```python
from build123d import *

# Parameters (mm, degrees)
SALIENTE_EXTRUIR1_DEPTH = 600
CROQUIS2_R              = 1.25
CORTAR_EXTRUIR1_DEPTH   = 41


with BuildPart() as part:
    # Croquis1 → Saliente-Extruir1 (new body)
    with BuildSketch(Plane(origin=(0, 0, 0), x_dir=(0, 0, -1), z_dir=(1, 0, 0))):
        Polygon((-20, 0), (20, 0), (20, 15), (18.5, 15), (-18.5, 15), (-20, 15), align=None)
    extrude(amount=SALIENTE_EXTRUIR1_DEPTH)

    # Croquis2 → Cortar-Extruir1 (cut, through all)
    with BuildSketch(Plane(origin=(0, 0, -20), x_dir=(-1, 0, 0), z_dir=(0, 0, -1))):
        with Locations((-25, 7.5)):
            Circle(CROQUIS2_R)
        with Locations((-93.75, 7.5)):
            Circle(CROQUIS2_R)
        with Locations((-162.5, 7.5)):
            Circle(CROQUIS2_R)
        with Locations((-231.25, 7.5)):
            Circle(CROQUIS2_R)
        with Locations((-368.75, 7.5)):
            Circle(CROQUIS2_R)
        with Locations((-437.5, 7.5)):
            Circle(CROQUIS2_R)
        with Locations((-506.25, 7.5)):
            Circle(CROQUIS2_R)
        with Locations((-575, 7.5)):
            Circle(CROQUIS2_R)
        with Locations((-300, 7.5)):
            Circle(CROQUIS2_R)
        Polygon((-600, 15), (-585, 15), (-600, 0), align=None)
        Polygon((0, 15), (-15, 15), (0, 0), align=None)
    extrude(amount=-CORTAR_EXTRUIR1_DEPTH, mode=Mode.SUBTRACT)


solid = part.part
```
Source: CAD feature listing. Evaluate the final solid. Frame: model axes, mm. Round coordinates to 2 decimals unless told otherwise and drop trailing zeros. Loops run counter-clockwise (first coordinate to the right, second up) from the corner with the lowest first, then second, coordinate; pieces in that order, holes last. Notation, with made-up numbers: M 29,-36.5 L 47,-36.5 A21 cw 47,-25.5 Z; hole C 66.5,61 d1. An arc over 180 degrees is marked long. Use a Markdown table: item, result. Add a question column.
1. Contact query for flat-ended pins moving along their axis: pin 1 (2 mm diameter, centred on x = 437.5, y = 7.5, fed in from -Z); pin 2 (4 mm diameter, centred on y = 5.5, z = -14.5, fed in from -X); pin 3 (8 mm diameter, centred on y = 11.5, z = 1.5, fed in from +X). Output: stop coordinate, or through.
2. Ray query, line 1 along Y through (x, z) = (575, -2); line 2 along Y through (x, z) = (93, 2); line 3 along X through (y, z) = (13.25, 2). Return the intervals inside material, ascending. Write a range as [from, to].
3. Cut plane A-A, the plane z = 3. State how many separate pieces and enclosed holes the cut face has, and give its area (3 significant figures).
4. Cut plane B-B, the plane y = 11.75. Output: boundary loops of the cut face in (x, z).
Solution:
| question | item | result |
|---|---|---|
| 1 | pin 1 | passes through |
| 1 | pin 2 | stops at x = 3.5 |
| 1 | pin 3 | stops at x = 592.5 |
| 2 | line 1 | y = [0, 6.25], [8.75, 15] |
| 2 | line 2 | y = [0, 6.5], [8.5, 15] |
| 2 | line 3 | x = [13.25, 586.75] |
| 3 | separate pieces | 1 |
| 3 | enclosed holes | 9 |
| 3 | area | 8,730 mm2 |
| 4 | outline | M 11.75,-20 L 588.25,-20 L 588.25,20 L 11.75,20 Z |
